Design review of the part built by this model. Coordinates are the model's own, in mm. A direction names the side the tool comes from. Coordinates: 2 decimals unless noted, no trailing zeros. Write each loop counter-clockwise with the first axis right and the second up, starting at its lowest first coordinate (ties: lowest second). Pieces come first, ordered by that corner, then holes. Notation, with made-up numbers: (34, 86.25) -> (91, 86.25) arc R19 cw to (91, 108.25) -> close; hole circle Ø11 at (27, 7.5). An arc over 180 degrees is marked (long way). One line per question, with ' | ' between items. Start each with the question number.
Q1. For P1, Ø21, axis at x = 64, y = 4.5, coming from the -Z side; P2, Ø12, axis at x = -15.5, z = 26, coming from the +Y side; P3, Ø16.5, axis at x = 5.5, y = -24, coming from the +Z side (3 decimals), all flat-tipped, find the tip position at first contact; note any pin that passes through.
Q2. Draft analysis for pull direction X (two halves, no side actions). For faces 5 (the flat face through (22.225, -17, 18)), 6 (the cylindrical face through (45.983, -0.356, 38.197)), 7 (the flat face through (1, -36, 9.525)), state which applies: pulls with the +X half, pulls with the -X half, needs draft (parallel to the pull), parting line crosses it, or undercut.
Q3. Add section A-A on x = 74. State the section outline as (y, z) points (3 decimals), and give its area (3 significant figures).
Q4. Add section B-B on y = -30.5. State the section outline as (x, z) points (3 decimals).
Q5. Wall thickness on probe 1 along Y at (x, z) = (20.5, 51); probe 2 along Z at (x, y) = (87.5, -2) (3 decimals); probe 3 along X at (y, z) = (20, 7) (3 decimals): over which ranges is each line inside the solid? List them lowest first.
Q6. For faces 1 (the flat face through (-3, -7.938, 30)), 2 (the flat face through (59, 0, 43.162)), 3 (the flat face through (41.275, -1, 4)), 4 (the flat face through (43, 25.4, 42)), list the 3-axis set-ups (+Z, -Z, +X, -X, +Y, -Y) from which the entire face can be reached by the end or side of a thin tool; tool diameter is ignored.
from build123d import *

# Parameters (mm, degrees)
F1_DEPTH = 63.5
F0_W     = 16.342798
F0_H     = 19.05
F2_DEPTH = 25.4
F3_DEPTH = 7.9375
F0_W_2   = 25.4
F0_H_2   = 28.575
F5_R     = 5.08


with BuildPart() as f1:
    # F0 (on Front) → F1 (new body, symmetric)
    with BuildSketch(Plane.XZ):
        Polygon((-41.275, -9.525), (41.275, -9.525), (41.275, 9.525), (22.225, 9.525), (-41.275, 9.525), align=None)
    extrude(amount=F1_DEPTH, both=True)

    # F0 (on Front) → F2 (join, symmetric)
    with BuildSketch(Plane.XZ):
        with BuildLine():
            Line((22.225, 9.525), (41.275, 9.525))
            Line((41.275, 9.525), (41.275, 26.651896))
            ThreePointArc((41.275, 26.651896), (46.110667, 38.326229), (57.785, 43.161896))
            Line((57.785, 43.161896), (60.325, 43.161896))
            Line((60.325, 43.161896), (60.325, 62.211896))
            Line((60.325, 62.211896), (57.785, 62.211896))
            add(Edge.make_bspline(
                [(55.339805, 62.127728), (56.163925, 62.171613), (56.97924, 62.199852), (57.785, 62.211896)],
                knots=[109.850246, 109.850246, 109.850246, 109.850246, 112.199789, 112.199789, 112.199789, 112.199789], degree=3))
            ThreePointArc((55.339805, 62.127728), (31.790147, 50.916711), (22.225, 26.651896))
            Line((22.225, 26.651896), (22.225, 9.525))
        make_face()
        with Locations((68.496399, 52.686896)):
            Rectangle(F0_W, F0_H)
    extrude(amount=F2_DEPTH, both=True)

    # F0 (on Front) → F3 (join, symmetric)
    with BuildSketch(Plane.XZ):
        with BuildLine():
            add(Edge.make_bspline(
                [(-41.275, 9.525), (-40.967457, 23.823205), (16.809013, 60.07592), (55.339805, 62.127728)],
                knots=[0, 0, 0, 0, 109.850246, 109.850246, 109.850246, 109.850246], degree=3))
            Line((-41.275, 9.525), (22.225, 9.525))
            Line((22.225, 9.525), (22.225, 26.651896))
            ThreePointArc((22.225, 26.651896), (31.790147, 50.916711), (55.339805, 62.127728))
        make_face()
    extrude(amount=F3_DEPTH, both=True)

    # F0 (on Front) → F4 (revolve)
    with BuildSketch(Plane.XZ):
        with Locations((98.425, 52.3875)):
            Rectangle(F0_W_2, F0_H_2)
    revolve(axis=Axis((85.725, 0, 52.187027), (0, 0, -1)))

    # F5
    f5_edges = [f1.edges().sort_by_distance(p)[0] for p in [
        (41.275, -63.5, 0),
        (41.275, 63.5, 0),
        (-41.275, -63.5, 0),
        (-41.275, 63.5, 0),
    ]]
    fillet(f5_edges, radius=F5_R)


solid = f1.part
Output values:
1) P1: stops at z = 38.1 | P2: stops at y = 7.94 | P3: stops at z = 9.525
2) face 5: pulls with the -X half | face 6: undercut | face 7: needs draft
3) outline: (-25.4, 43.162) -> (-22.532, 43.162) -> (-22.532, 38.1) -> (22.532, 38.1) -> (22.532, 43.162) -> (25.4, 43.162) -> (25.4, 62.212) -> (22.532, 62.212) -> (22.532, 66.675) -> (-22.532, 66.675) -> (-22.532, 62.212) -> (-25.4, 62.212) -> close | area: 1,400 mm2
4) outline: (-41.275, -9.525) -> (41.275, -9.525) -> (41.275, 9.525) -> (-41.275, 9.525) -> close
5) probe 1: y = -7.94 to 7.94 | probe 2: z = 38.1 to 66.675 | probe 3: x = -41.275 to 41.275
6) face 1: +Z, -X, -Y | face 2: -Z | face 3: -Z, +X, +Y, -Y | face 4: +Z, +X, -X, +Y
